```python
from build123d import *

# Parameters (mm, degrees)
SKETCH1_R           = 6.35
BOSS_EXTRUDE1_DEPTH = 12.7
CUT_EXTRUDE1_DEPTH  = 16.554259867


with BuildPart() as part:
    # Sketch1 → Boss-Extrude1 (new body)
    with BuildSketch(Plane(origin=(0, 0, 0), x_dir=(1, 0, 0), z_dir=(0, 1, 0))):
        with Locations(Location((0, 0, 0), (0, 0, 270))):
            Circle(SKETCH1_R)
        with BuildLine():
            Line((1.397, 1.722711816), (1.397, -1.722711816))
            ThreePointArc((1.397, -1.722711816), (-4.445, 0), (1.397, 1.722711816))
        make_face(mode=Mode.SUBTRACT)
    extrude(amount=BOSS_EXTRUDE1_DEPTH)

    # Sketch2 → Cut-Extrude1 (cut, through all)
    with BuildSketch(Plane(origin=(0, 12.7, 0), x_dir=(1, 0, 0), z_dir=(0, 1, 0))):
        with BuildLine():
            Line((-0.882804878, 3.151302102), (-0.882804878, -3.151302102))
            ThreePointArc((-0.882804878, -3.151302102), (0.65244788, -3.06792374), (1.397, -1.722711816))
            Line((1.397, -1.722711816), (1.397, 1.722711816))
            ThreePointArc((1.397, 1.722711816), (0.65244788, 3.06792374), (-0.882804878, 3.151302102))
        make_face()
    extrude(amount=-CUT_EXTRUDE1_DEPTH, mode=Mode.SUBTRACT)


solid = part.part
```
Input: part model. Units: mm. Frame: model coordinates. A direction names the side the tool comes from. Give positions to 0.01 mm unless a question says otherwise; leave off trailing zeros. Order: outer loops, then holes, each group sorted by start corner. A loop starts at its lowest first (then second) coordinate and runs counter-clockwise, first axis right, second up.
1. Pin query (flat end, axial travel): pin 1 Ø4 at (y, z) = (2.5, -2.5) entering from -X; pin 2 Ø2 at (x, y) = (3, 6.5) entering from -Z; pin 3 Ø1 at (y, z) = (4, 1.5) entering from +X. Return the tip coordinate at first contact, or that it passes through.
Computed:
pin 1: stops at x = -6.33
pin 2: stops at z = -6.03
pin 3: stops at x = 6.27
2. Line query: probe 1 along X at (y, z) = (9.75, 0) (3 decimals); probe 2 along Z at (x, y) = (-1.27, 5.25) (3 decimals); probe 3 along X at (y, z) = (9.5, -1.25). Output: solid intervals per line, ascending.
Computed:
probe 1: x = -6.35 to -4.445, 1.397 to 6.35
probe 2: z = -6.222 to -3.175, 3.175 to 6.222
probe 3: x = -6.23 to -4.19, 1.4 to 6.23
3. Cut plane D-D (x = 3.25). Return loops of the section in (y, z), and give its area (3 significant figures).
Computed:
outline: (0, -5.46) - (12.7, -5.46) - (12.7, 5.46) - (0, 5.46) - close
area: 139 mm2
4. Cut plane B-B (x = 0). Return loops of the section in (y, z), and give its area (3 significant figures).
Computed:
outline: (0, -6.35) - (12.7, -6.35) - (12.7, -3.3) - (0, -3.3) - close; (0, 3.3) - (12.7, 3.3) - (12.7, 6.35) - (0, 6.35) - close
area: 77.5 mm2
5. Draft query along X for faces 3 (the face through (-3.86, 6.26, -5.04)), 4 (the face through (2, 0, 0)), 5 (the face through (0.671, 6.439, -3.056)). Return one class per face: released by +X, released by -X, zero draft, split by the parting line, or undercut.
Computed:
face 3: split by the parting line
face 4: zero draft
face 5: undercut
6. Set-up query: faces 1 (the face through (1.397, 6, 0)), 2 (the face through (2, 12.7, 0)). Return all of +Z, -Z, +X, -X, +Y, -Y with unobstructed straight access to the full face (end or side cutting, diameter ignored); none if empty.
Computed:
face 1: +Y, -Y
face 2: +Z, -Z, +X, -X, +Y
7. Cut plane A-A (z = 0). Return loops of the section in (x, y) (3 decimals).
Computed:
outline: (-6.35, 0) - (-4.445, 0) - (-4.445, 12.7) - (-6.35, 12.7) - close; (1.397, 0) - (6.35, 0) - (6.35, 12.7) - (1.397, 12.7) - close
